Check sheet for the modelled part. Datum: model origin and axes. Units: mm. Face numbers are marked on the shaded views. A direction names the side the tool comes from. Round coordinates to 2 decimals unless told otherwise and drop trailing zeros. Loops run counter-clockwise (first coordinate to the right, second up) from the corner with the lowest first, then second, coordinate; pieces in that order, holes last. Notation, with made-up numbers: (-16, -25.75) - (41, -25.75) arc R14 cw to (41, -7.75) - close; hole circle Ø11 at (52, 84.25). An arc over 180 degrees is marked (long way). Answer in a Markdown table with one row per item. Add a question column.
(1) Cross-section at C-C on y = 22. Enter the section's corners in (x, z), then the cut area to 3 significant figures.
(2) Thickness scan on line 1 along X through (y, z) = (6, -20.5); line 2 along Z through (x, y) = (3, 16.5); line 3 along Y through (x, z) = (40, -14). Record the ranges inside material, lowest first.
(3) Mould release check, pull along Z, two halves, no side actions. Record for the marked faces 1, 2, 3 and 4: +Z half, -Z half, draft (parallel to the pull), parting line (faces both ways), or undercut.
(4) Access from +Z, -Z, +X, -X, +Y, -Y to the whole of each face (thin tool, end or side, straight path). Record for the marked faces 5 and 6.
(5) Gauge pin test, flat ends, axial feed: pin 1 (1 mm diameter, centred on x = 71, z = -8.5, fed in from -Y); pin 2 (3.5 mm diameter, centred on x = 46, z = -32, fed in from +Y); pin 3 (0.9 mm diameter, centred on x = -2, y = 38.5, fed in from -Z); pin 4 (3.5 mm diameter, centred on x = 73.5, z = -31, fed in from +Y). Record the tip position at first contact, or that the pin passes through.
(6) Cross-section at D-D on y = 32.5. Enter the section's corners in (x, z), then the cut area to 3 significant figures.
(7) Cross-section at B-B on x = 26. Enter the section's corners in (y, z).
(8) Cross-section at A-A on z = -24.5. Enter the section's corners in (x, y), then the cut area to 3 significant figures.
from build123d import *

# Parameters (mm, degrees)
SKETCH1_W           = 83
SKETCH1_H           = 36
SKETCH1_W_2         = 77
SKETCH1_H_2         = 30
BOSS_EXTRUDE1_DEPTH = 5
BOSS_EXTRUDE2_DEPTH = 40
SKETCH3_W           = 83
SKETCH3_H           = 36
BOSS_EXTRUDE3_DEPTH = 1
SKETCH4_W           = 9.752325518
SKETCH4_H           = 10
CUT_EXTRUDE1_DEPTH  = 15
CUT_EXTRUDE2_REACH  = 100.595
SKETCH5_W           = 7.400592898
SKETCH5_H           = 21.28859468


with BuildPart() as part:
    # Sketch1 → Boss-Extrude1 (new body)
    with BuildSketch(Plane(origin=(0, 0, 0), x_dir=(1, 0, 0), z_dir=(0, 1, 0))):
        with Locations((38.5, 15)):
            Rectangle(SKETCH1_W, SKETCH1_H)
        with Locations((38.5, 15)):
            Rectangle(SKETCH1_W_2, SKETCH1_H_2, mode=Mode.SUBTRACT)
    extrude(amount=BOSS_EXTRUDE1_DEPTH)

    # Sketch2 → Boss-Extrude2 (add)
    with BuildSketch(Plane(origin=(0, 5, 0), x_dir=(1, 0, 0), z_dir=(0, 1, 0))):
        Polygon((80, -3), (80, 33), (70.247674482, 33), (70.247674482, 30), (77, 30), (77, 0), (0, 0), (0, 30), (6.752325518, 30), (6.752325518, 33), (-3, 33), (-3, -3), align=None)
    extrude(amount=BOSS_EXTRUDE2_DEPTH)

    # Sketch3 → Boss-Extrude3 (add)
    with BuildSketch(Plane.XZ):
        with Locations((38.5, -15)):
            Rectangle(SKETCH3_W, SKETCH3_H)
    extrude(amount=-BOSS_EXTRUDE3_DEPTH)

    # Sketch4 → Cut-Extrude1 (cut)
    with BuildSketch(Plane(origin=(0, 0, -33), x_dir=(-1, 0, 0), z_dir=(0, 0, -1))):
        with Locations((-1.876162759, 40)):
            Rectangle(SKETCH4_W, SKETCH4_H)
    extrude(amount=-CUT_EXTRUDE1_DEPTH, mode=Mode.SUBTRACT)

    # Sketch5 → Cut-Extrude2 (cut, up to next)
    with BuildSketch(Plane(origin=(0, 0, -33), x_dir=(-1, 0, 0), z_dir=(0, 0, -1)), mode=Mode.PRIVATE) as cut_extrude2_sk1:
        with Locations((-73.299703551, 35.04429734)):
            Rectangle(SKETCH5_W, SKETCH5_H)
    cut_extrude2_tool1 = extrude(cut_extrude2_sk1.sketch, amount=-CUT_EXTRUDE2_REACH, mode=Mode.PRIVATE) & part.part
    add(cut_extrude2_tool1.solids().sort_by_distance((73.299704, 35.044297, -33))[0], mode=Mode.SUBTRACT)


solid = part.part
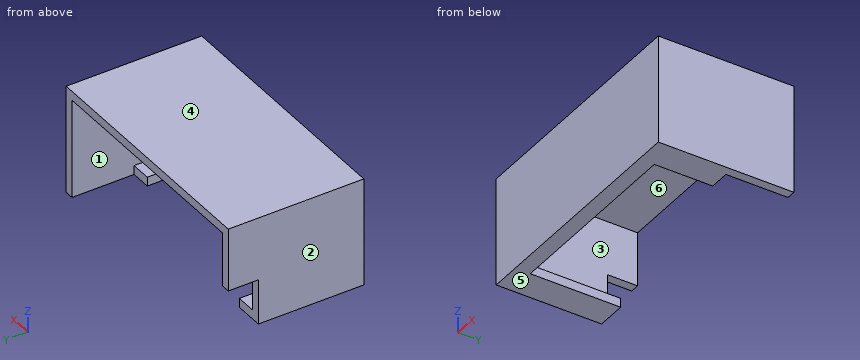
Answers:
| question | item | result |
|---|---|---|
| 1 | outline | (-3, -33) - (6.75, -33) - (6.75, -30) - (0, -30) - (0, 0) - (77, 0) - (77, -30) - (70.25, -30) - (70.25, -33) - (80, -33) - (80, 3) - (-3, 3) - close |
| 1 | area | 488 mm^2 |
| 2 | line 1 | x = -3 to 0, 77 to 80 |
| 2 | line 2 | z = -33 to -30, 0 to 3 |
| 2 | line 3 | y = 0 to 1 |
| 3 | face 1 | undercut |
| 3 | face 2 | draft |
| 3 | face 3 | undercut |
| 3 | face 4 | +Z half |
| 4 | face 5 | -Z, +X, -X, +Y, -Y |
| 4 | face 6 | +Y |
| 5 | pin 1 | stops at y = 0 |
| 5 | pin 2 | stops at y = 5 |
| 5 | pin 3 | stops at z = -18 |
| 5 | pin 4 | stops at y = 24.4 |
| 6 | outline | (-3, -33) - (6.75, -33) - (6.75, -30) - (0, -30) - (0, 0) - (77, 0) - (77, -33) - (80, -33) - (80, 3) - (-3, 3) - close |
| 6 | area | 467 mm^2 |
| 7 | outline | (0, -33) - (5, -33) - (5, -30) - (1, -30) - (1, 0) - (45, 0) - (45, 3) - (0, 3) - close |
| 8 | outline | (-3, 0) - (80, 0) - (80, 45) - (77, 45) - (77, 1) - (0, 1) - (0, 35) - (-3, 35) - close |
| 8 | area | 317 mm^2 |
